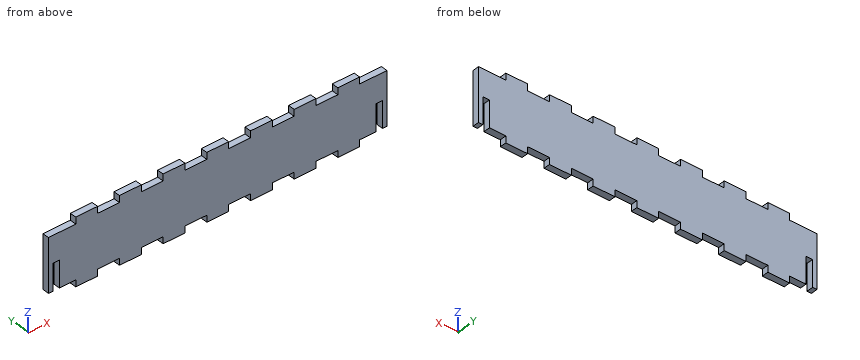
```python
from build123d import *

# Parameters (mm, degrees)
F0_W     = 145
F0_H     = 30
F1_DEPTH = 3
F2_W     = 10
F2_H     = 3
F3_DEPTH = 25
F4_DEPTH = 5
F5_DEPTH = 5
F6_W     = 3
F6_H     = 12
F7_DEPTH = 25


with BuildPart() as f1:
    # F0 (on Front) → F1 (new body)
    with BuildSketch(Plane.XZ):
        Rectangle(F0_W, F0_H)
    extrude(amount=F1_DEPTH)

    # F2 (on face) → F3 (cut)
    with BuildSketch(Plane.XZ.offset(3)):
        with Locations((-70, -13.5)):
            Rectangle(F2_W, F2_H)
        with Locations((-70, 13.5)):
            Rectangle(F2_W, F2_H)
        with Locations((-50, -13.5)):
            Rectangle(F2_W, F2_H)
        with Locations((-50, 13.5)):
            Rectangle(F2_W, F2_H)
        with Locations((-30, -13.5)):
            Rectangle(F2_W, F2_H)
        with Locations((-30, 13.5)):
            Rectangle(F2_W, F2_H)
        with Locations((-10, -13.5)):
            Rectangle(F2_W, F2_H)
        with Locations((-10, 13.5)):
            Rectangle(F2_W, F2_H)
        with Locations((10, -13.5)):
            Rectangle(F2_W, F2_H)
        with Locations((10, 13.5)):
            Rectangle(F2_W, F2_H)
        with Locations((30, -13.5)):
            Rectangle(F2_W, F2_H)
        with Locations((30, 13.5)):
            Rectangle(F2_W, F2_H)
        with Locations((50, -13.5)):
            Rectangle(F2_W, F2_H)
        with Locations((50, 13.5)):
            Rectangle(F2_W, F2_H)
        with Locations((70, -13.5)):
            Rectangle(F2_W, F2_H)
        with Locations((70, 13.5)):
            Rectangle(F2_W, F2_H)
    extrude(amount=-F3_DEPTH, mode=Mode.SUBTRACT)

    # F4 (add): faces of the model
    f4_faces = [f1.faces().sort_by_distance(p)[0] for p in [
        (72.5, -1.5, 0),
        (-72.5, -1.5, 0),
    ]]
    extrude(f4_faces, amount=F4_DEPTH, dir=(1, 0, 0))

    # F5 (add): a face of the model
    f5_faces = [f1.faces().sort_by_distance(p)[0] for p in [
        (-72.5, -1.5, 0),
    ]]
    extrude(f5_faces, amount=F5_DEPTH)

    # F6 (on face) → F7 (cut)
    with BuildSketch(Plane(origin=(0, 0, 0), x_dir=(-1, 0, 0), z_dir=(0, 1, 0))):
        with Locations((-74, -6)):
            Rectangle(F6_W, F6_H)
        with Locations((74, -6)):
            Rectangle(F6_W, F6_H)
    extrude(amount=-F7_DEPTH, mode=Mode.SUBTRACT)


solid = f1.part
```
For this review, take the finished solid that the model builds, in its own axes (mm). Round coordinates to 2 decimals unless told otherwise and drop trailing zeros. Write each loop counter-clockwise with the first axis right and the second up, starting at its lowest first coordinate (ties: lowest second). Pieces come first, ordered by that corner, then holes. Notation, with made-up numbers: (-17, 49) -> (-4, 49) arc R32 ccw to (-4, 85) -> close; hole circle Ø4 at (86, -20.5). An arc over 180 degrees is marked (long way). Use one line per item in the form item = value.
Q1. Clearance check with flat-ended pins moving along their axes: pin 1 Ø0.9 at (y, z) = (-1, 13) entering from +X; pin 2 Ø0.9 at (x, y) = (8.5, -2) entering from +Z; pin 3 Ø1.5 at (x, y) = (70, -2) entering from -Z. State where each tip first meets the part, or that it passes through.
Resolved:
pin_1 = 65
pin_2 = 12
pin_3 = -12
Q2. To check wall thickness, follow probe 1 along X at (y, z) = (-1.65, -0.75); probe 2 along Z at (x, y) = (-26.5, -1.2). State the ranges of each line that lie inside material, in increasing order. Write a range as from..to.
Resolved:
probe_1 = -77.5..-75.5, -72.5..72.5, 75.5..77.5
probe_2 = -12..12
Q3. Consider section A-A (z = -2.5). State the section outline as (x, y) points.
Resolved:
outline = (-77.5, -3) -> (-75.5, -3) -> (-75.5, 0) -> (-77.5, 0) -> close; (-72.5, -3) -> (72.5, -3) -> (72.5, 0) -> (-72.5, 0) -> close; (75.5, -3) -> (77.5, -3) -> (77.5, 0) -> (75.5, 0) -> close
Q4. Consider section B-B (x = 51.5). State the section outline as (y, z) points.
Resolved:
outline = (-3, -12) -> (0, -12) -> (0, 12) -> (-3, 12) -> close
